Geometry check sheet. Reference: the model listing, model coordinates, mm. A direction names the side the tool comes from. Coordinates: 2 decimals unless noted, no trailing zeros. Loops run counter-clockwise (first coordinate to the right, second up) from the corner with the lowest first, then second, coordinate; pieces in that order, holes last. Notation, with made-up numbers: (24, 27) -> (61, 27) arc R24 ccw to (61, 47) -> close; hole circle Ø7 at (39.5, -15.75). An arc over 180 degrees is marked (long way). Answer as a JSON object with one key per item and string values.
from build123d import *

# Parameters (mm, degrees)
SKETCH2_R                = 15.5
SKETCH2_R_2              = 1.75
SKETCH2_R_3              = 7.5
FLANGE_DEPTH             = 15
SKETCH3_R                = 8.5
O_RING_SEAT_DEPTH        = 0.5
SKETCH5_R                = 1
OUTLET_DEPTH             = 27.561249971
BOSS_EXTRUDE2_REACH      = 39.766
BOSS_EXTRUDE2_END_RADIUS = 15.5
SKETCH6_R                = 3
SKETCH6_R_2              = 1


with BuildPart() as part:
    # Sketch2 → Flange (new body)
    with BuildSketch(Plane(origin=(0, 0, 0), x_dir=(0, 0, -1), z_dir=(1, 0, 0))):
        Circle(SKETCH2_R)
        with Locations((0, 12)):
            Circle(SKETCH2_R_2, mode=Mode.SUBTRACT)
        with Locations((12, 0)):
            Circle(SKETCH2_R_2, mode=Mode.SUBTRACT)
        with Locations((0, -12)):
            Circle(SKETCH2_R_2, mode=Mode.SUBTRACT)
        with Locations((-12, 0)):
            Circle(SKETCH2_R_2, mode=Mode.SUBTRACT)
        Circle(SKETCH2_R_3, mode=Mode.SUBTRACT)
    extrude(amount=FLANGE_DEPTH)

    # Sketch3 → O-Ring Seat (cut)
    with BuildSketch(Plane(origin=(15, 0, 0), x_dir=(0, 0, -1), z_dir=(1, 0, 0))):
        Circle(SKETCH3_R)
    o_ring_seat = extrude(amount=-O_RING_SEAT_DEPTH, mode=Mode.SUBTRACT)

    # Mirror1: O-Ring Seat across plane
    add(o_ring_seat.mirror(Plane.ZY.offset(-7.5)), mode=Mode.SUBTRACT)

    # Sketch5 → Outlet (cut, through all)
    with BuildSketch(Plane(origin=(0, 0, 0), x_dir=(1, 0, 0), z_dir=(0, 1, 0))):
        with Locations(Location((7.5, 6.5, 0), (0, 0, 90))):
            Circle(SKETCH5_R)
    outlet = extrude(amount=OUTLET_DEPTH, mode=Mode.SUBTRACT)

    # Boss-Extrude2: up to this cylinder (the profile starts outside it)
    boss_extrude2_end = Plane(origin=(7.5, 0, 0), z_dir=(-1, 0, 0)) * Cylinder(BOSS_EXTRUDE2_END_RADIUS, 111.532, mode=Mode.PRIVATE)
    # Sketch6 → Boss-Extrude2 (add, up to the surface)
    with BuildSketch(Plane(origin=(0, 15.5, 0), x_dir=(1, 0, 0), z_dir=(0, 1, 0)), mode=Mode.PRIVATE) as boss_extrude2_sk1:
        with Locations(Location((7.5, 6.5, 0), (0, 0, 270))):
            Circle(SKETCH6_R)
        with Locations(Location((7.5, 6.5, 0), (0, 0, 90))):
            Circle(SKETCH6_R_2, mode=Mode.SUBTRACT)
    boss_extrude2_tool1 = extrude(boss_extrude2_sk1.sketch, amount=-BOSS_EXTRUDE2_REACH, mode=Mode.PRIVATE) - boss_extrude2_end
    boss_extrude2 = boss_extrude2_tool1.solids().sort_by_distance((7.5, 15.5, -9.415147))[0]
    add(boss_extrude2)

    # Inlet: Outlet, Boss-Extrude2 across plane
    add(outlet.mirror(Plane.XY), mode=Mode.SUBTRACT)
    add(boss_extrude2.mirror(Plane.XY))


solid = part.part
1. Tool access check on faces 1 (the face through (15, -7, -7)), 2 (the face through (0.246, 7.167, -4.57)), 3 (the face through (14.5, -8, 0)). Record the directions out of +Z, -Z, +X, -X, +Y, -Y that give a thin tool (end or side, any length) a straight path to the whole face; none if there is none.
Evaluation:
{"face 1": "+Z, -Z, +X, +Y, -Y", "face 2": "-X", "face 3": "+X"}
2. Depth check by flat-ended pin: P1, Ø3, axis at y = 12, z = 0, coming from the -X side; P2, Ø15.5, axis at y = 0, z = 0, coming from the +X side; P3, Ø8, axis at x = 6, z = 11, coming from the -Y side; P4, Ø3, axis at x = 9.5, y = -5, coming from the +Z side. Enter the tip coordinate at first touch or a pass-through.
Evaluation:
{"P1": "passes through", "P2": "stops at x = 14.5", "P3": "stops at y = -13.83", "P4": "stops at z = 15.1"}
3. Mould release check, pull along Y, two halves, no side actions. Record for faces 4 (the face through (7.4, -9.43, 12.3)), 5 (the face through (0, -7, -7)), 6 (the face through (7.395, 0.526, 10.331)), 7 (the face through (7.395, 13.735, 0.228)): released by +Y, released by -Y, zero draft, split by the parting line, or undercut.
Evaluation:
{"face 4": "split by the parting line", "face 5": "zero draft", "face 6": "undercut", "face 7": "undercut"}
4. Section check B-B, the plane z = 0. Record the boundary of the cut face in (x, y), then the cut area to 3 significant figures.
Evaluation:
{"outline": "(0, -15.5) -> (15, -15.5) -> (15, -13.75) -> (0, -13.75) -> close; (0, -10.25) -> (15, -10.25) -> (15, -8.5) -> (14.5, -8.5) -> (14.5, -7.5) -> (0.5, -7.5) -> (0.5, -8.5) -> (0, -8.5) -> close; (0, 8.5) -> (0.5, 8.5) -> (0.5, 7.5) -> (14.5, 7.5) -> (14.5, 8.5) -> (15, 8.5) -> (15, 10.25) -> (0, 10.25) -> close; (0, 13.75) -> (15, 13.75) -> (15, 15.5) -> (0, 15.5) -> close", "area": "133 mm^2"}
5. Section check A-A, the plane x = 7.5. Record the boundary of the cut face in (y, z), then the cut area to 3 significant figures.
Evaluation:
{"outline": "(0, -7.5) arc R7.5 cw to (0, 7.5) -> (15.5, 7.5) -> (15.5, 9.5) -> (12.25, 9.5) arc R15.5 ccw (long way) to (12.25, -9.5) -> (15.5, -9.5) -> (15.5, -7.5) -> close; (5.1, -5.5) -> (15.5, -5.5) -> (15.5, -3.5) -> (15.1, -3.5) arc R15.5 ccw to (15.1, 3.5) -> (15.5, 3.5) -> (15.5, 5.5) -> (5.1, 5.5) arc R7.5 cw to start; hole circle Ø3.5 at (-12, 0); hole circle Ø3.5 at (0, -12); hole circle Ø3.5 at (0, 12); hole circle Ø3.5 at (12, 0)", "area": "510 mm^2"}
6. Thickness scan on probe 1 along Y at (x, z) = (9, 0); probe 2 along Y at (x, z) = (14.8, 0); probe 3 along X at (y, z) = (8.5, 6.5). Record the ranges inside material, lowest first. Write a range as from..to.
Evaluation:
{"probe 1": "y = -15.5..-13.75, -10.25..-7.5, 7.5..10.25, 13.75..15.5", "probe 2": "y = -15.5..-13.75, -10.25..-8.5, 8.5..10.25, 13.75..15.5", "probe 3": "x = 0..6.5, 8.5..15"}
7. Section check C-C, the plane y = 7. Record the boundary of the cut face in (x, z), then the cut area to 3 significant figures.
Evaluation:
{"outline": "(0, -13.83) -> (15, -13.83) -> (15, -4.82) -> (14.5, -4.82) -> (14.5, -2.69) -> (0.5, -2.69) -> (0.5, -4.82) -> (0, -4.82) -> close; (0, 4.82) -> (0.5, 4.82) -> (0.5, 2.69) -> (14.5, 2.69) -> (14.5, 4.82) -> (15, 4.82) -> (15, 13.83) -> (0, 13.83) -> close; hole circle Ø2 at (7.5, -6.5); hole circle Ø2 at (7.5, 6.5)", "area": "324 mm^2"}
8. Section check D-D, the plane z = -6.5. Record the boundary of the cut face in (x, y).
Evaluation:
{"outline": "(0, -14.07) -> (15, -14.07) -> (15, -5.48) -> (14.5, -5.48) -> (14.5, -3.74) -> (0.5, -3.74) -> (0.5, -5.48) -> (0, -5.48) -> close; (0, 5.48) -> (0.5, 5.48) -> (0.5, 3.74) -> (6.5, 3.74) -> (6.5, 15.5) -> (4.5, 15.5) -> (4.5, 14.07) -> (0, 14.07) -> close; (8.5, 3.74) -> (14.5, 3.74) -> (14.5, 5.48) -> (15, 5.48) -> (15, 14.07) -> (10.5, 14.07) -> (10.5, 15.5) -> (8.5, 15.5) -> close"}
